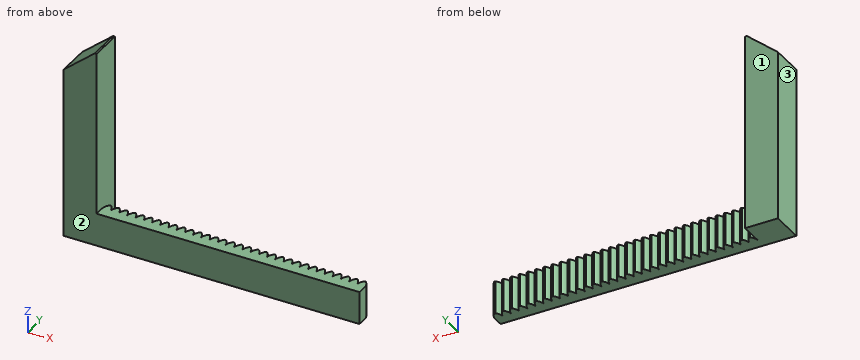
```python
from build123d import *

# Parameters (mm, degrees)
BOSS_EXTRUDE1_DEPTH = 10
CUT_EXTRUDE4_DEPTH  = 10
LPATTERN2_COUNT     = 32
LPATTERN2_PITCH     = 2.5


with BuildPart() as part:
    # Sketch1 → Boss-Extrude1 (new body)
    with BuildSketch(Plane(origin=(0, 0, 0), x_dir=(1, 0, 0), z_dir=(0, 1, 0))):
        Polygon((-50, -47.085841971), (-40.568273737, -55), (-40, -55), (-40, -5), (40, -5), (40, 5), (-40, 5), (-50, 5), align=None)
    extrude(amount=BOSS_EXTRUDE1_DEPTH)

    # Sketch5 → Cut-Extrude4 (cut)
    with BuildSketch(Plane.XY.offset(5)):
        with BuildLine():
            Line((40, 10), (37.5, 10))
            Line((37.5, 10), (37.5, 3.221403126))
            ThreePointArc((37.5, 3.221403126), (37.853347708, 4.366700719), (38.55, 5.342014394))
            Line((38.55, 5.342014394), (38.95, 5.342014394))
            ThreePointArc((38.95, 5.342014394), (39.646652292, 4.366700719), (40, 3.221403126))
            Line((40, 3.221403126), (40, 10))
        make_face()
    cut_extrude4 = extrude(amount=-CUT_EXTRUDE4_DEPTH, mode=Mode.SUBTRACT)

    # LPattern2: Cut-Extrude4 ×32
    with Locations(*[(-i * LPATTERN2_PITCH, 0, 0) for i in range(1, LPATTERN2_COUNT)]):
        add(cut_extrude4, mode=Mode.SUBTRACT)


solid = part.part
```
Here's how the part is built. I have some questions about the finished solid (model axes, mm). Face numbers are marked on the shaded views. Coordinates: 2 decimals unless noted, no trailing zeros. Order: outer loops, then holes, each group sorted by start corner. A loop starts at its lowest first (then second) coordinate and runs counter-clockwise, first axis right, second up. Notation, with made-up numbers: (-12.75, -37) -> (21.25, -37) arc R16 ccw to (21.25, -23) -> close; hole circle Ø7 at (-22, 8.5). An arc over 180 degrees is marked (long way). Return JSON: item names as keys, results as strings.
1) If we section it at C-C on y = 8.25: List the corners of the cut face in (x, z) for me, plus the area to 3 significant figures.
Conclusion:
{"outline": "(-50, -5) -> (-40, -5) -> (-40, 55) -> (-40.57, 55) -> (-50, 47.09) -> close", "area": "563 mm²"}
2) I'm going to push flat-ended pins straight in: P1, Ø6, axis at x = 15.5, y = 2, coming from the +Z side; P2, Ø5, axis at y = 7, z = 27.5, coming from the +X side; P3, Ø1, axis at x = -4, z = 1.5, coming from the +Y side. Where does each tip first touch, or does it pass through?
Conclusion:
{"P1": "stops at z = 5", "P2": "stops at x = -40", "P3": "stops at y = 5.34"}
3) If we section it at A-A on y = 2.25: List the corners of the cut face in (x, z) for me.
Conclusion:
{"outline": "(-50, -5) -> (40, -5) -> (40, 5) -> (-40, 5) -> (-40, 55) -> (-40.57, 55) -> (-50, 47.09) -> close"}
4) If I drill on probe 1 along X at (y, z) = (9.5, 34.5); probe 2 along Z at (x, y) = (-1, 4.5); probe 3 along Y at (x, z) = (14, -0.5), over which ranges is the centre line in solid material (lowest first)?
Conclusion:
{"probe 1": "x = -50 to -40", "probe 2": "z = -5 to 5", "probe 3": "y = 0 to 5.29"}
5) Thinking about a two-plate mould opening in Y: for the marked faces 1, 2 and 3, which applies, +Y half, -Y half, draft (parallel to the pull), parting line (faces both ways), or undercut?
Conclusion:
{"face 1": "+Y half", "face 2": "-Y half", "face 3": "draft"}
6) If we section it at B-B on z = 33.5: List the corners of the cut face in (x, y) for me.
Conclusion:
{"outline": "(-50, 0) -> (-40, 0) -> (-40, 10) -> (-50, 10) -> close"}
7) If we section it at D-D on x = -44: List the corners of the cut face in (y, z) for me.
Conclusion:
{"outline": "(0, -5) -> (10, -5) -> (10, 52.12) -> (0, 52.12) -> close"}
